```python
from build123d import *

# Parameters (mm, degrees)
SKETCH1_W           = 100
SKETCH1_H           = 20
BOSS_EXTRUDE1_DEPTH = 7
SKETCH2_W           = 16
SKETCH2_H           = 8.428142516
CUT_EXTRUDE1_DEPTH  = 101
SKETCH3_W           = 100
SKETCH3_H           = 62
BOSS_EXTRUDE2_DEPTH = 30
SKETCH4_W           = 88
SKETCH4_H           = 56.5
CUT_EXTRUDE2_DEPTH  = 27.5
SKETCH5_W           = 7.686328358
SKETCH5_H           = 52.5
CUT_EXTRUDE3_DEPTH  = 7
SKETCH6_W           = 27.5
SKETCH6_H           = 13
CUT_EXTRUDE4_DEPTH  = 3
SKETCH7_W           = 58
SKETCH7_H           = 2.3
CUT_EXTRUDE5_DEPTH  = 23
CUT_EXTRUDE6_DEPTH  = 23
SKETCH10_W          = 78.288889142
SKETCH10_H          = 1.311621563
CUT_EXTRUDE7_DEPTH  = 2
FILLET2_R           = 5


with BuildPart() as part:
    # Sketch1 → Boss-Extrude1 (new body)
    with BuildSketch(Plane(origin=(0, 0, 0), x_dir=(1, 0, 0), z_dir=(0, 1, 0))):
        with Locations((-50, 10)):
            Rectangle(SKETCH1_W, SKETCH1_H)
    extrude(amount=BOSS_EXTRUDE1_DEPTH)

    # Sketch2 → Cut-Extrude1 (cut, through all)
    with BuildSketch(Plane.ZY.offset(100)):
        with Locations((-10, 0)):
            Rectangle(SKETCH2_W, SKETCH2_H)
    extrude(amount=-CUT_EXTRUDE1_DEPTH, mode=Mode.SUBTRACT)

    # Sketch3 → Boss-Extrude2 (add)
    with BuildSketch(Plane(origin=(0, 0, -20), x_dir=(-1, 0, 0), z_dir=(0, 0, -1))):
        with Locations((50, -24)):
            Rectangle(SKETCH3_W, SKETCH3_H)
    extrude(amount=BOSS_EXTRUDE2_DEPTH)

    # Sketch4 → Cut-Extrude2 (cut)
    with BuildSketch(Plane(origin=(0, 0, -50), x_dir=(-1, 0, 0), z_dir=(0, 0, -1))):
        with Locations((50, -24)):
            Rectangle(SKETCH4_W, SKETCH4_H)
    extrude(amount=-CUT_EXTRUDE2_DEPTH, mode=Mode.SUBTRACT)

    # Sketch5 → Cut-Extrude3 (cut, through all)
    with BuildSketch(Plane(origin=(-94, 0, 0), x_dir=(0, 0, -1), z_dir=(1, 0, 0))):
        with Locations((35.043164179, -24)):
            Rectangle(SKETCH5_W, SKETCH5_H)
    extrude(amount=-CUT_EXTRUDE3_DEPTH, mode=Mode.SUBTRACT)

    # Sketch6 → Cut-Extrude4 (cut)
    with BuildSketch(Plane.ZY.offset(6)):
        with Locations((-36.25, -24)):
            Rectangle(SKETCH6_W, SKETCH6_H)
    extrude(amount=-CUT_EXTRUDE4_DEPTH, mode=Mode.SUBTRACT)

    # Sketch7 → Cut-Extrude5 (cut)
    with BuildSketch(Plane(origin=(0, 0, -50), x_dir=(-1, 0, 0), z_dir=(0, 0, -1))):
        with Locations((35, -53.4)):
            Rectangle(SKETCH7_W, SKETCH7_H)
    extrude(amount=-CUT_EXTRUDE5_DEPTH, mode=Mode.SUBTRACT)

    # Sketch9 → Cut-Extrude6 (cut)
    with BuildSketch(Plane(origin=(0, -52.25, 0), x_dir=(1, 0, 0), z_dir=(0, 1, 0))):
        Polygon((-37.960647242, 38.5), (-64, 38.5), (-64, 33.5), (-37.960647242, 33.5), (-6.413001969, 33.5), (-6.413001969, 38.5), align=None)
    extrude(amount=-CUT_EXTRUDE6_DEPTH, mode=Mode.SUBTRACT)

    # Sketch10 → Cut-Extrude7 (cut)
    with BuildSketch(Plane(origin=(0, 7, 0), x_dir=(1, 0, 0), z_dir=(0, 1, 0))):
        with Locations((-50, 46.502804438)):
            Rectangle(SKETCH10_W, SKETCH10_H)
    cut_extrude7 = extrude(amount=-CUT_EXTRUDE7_DEPTH, mode=Mode.SUBTRACT)

    # Mirror1: Cut-Extrude7 across plane
    add(cut_extrude7.mirror(Plane.ZX.offset(-24)), mode=Mode.SUBTRACT)

    # Fillet2
    fillet2_edges = [part.edges().sort_by_distance(p)[0] for p in [
        (-50, 7, 0),
    ]]
    fillet(fillet2_edges, radius=FILLET2_R)


solid = part.part
```
Part model, mm, in its own coordinate system. A direction names the side the tool comes from. Round coordinates to 2 decimals unless told otherwise and drop trailing zeros. Order: outer loops, then holes, each group sorted by start corner. A loop starts at its lowest first (then second) coordinate and runs counter-clockwise, first axis right, second up. Notation, with made-up numbers: M -14,-26 L 30,-26 A9 cw 30,-11 Z; hole C -12,-20 d3. An arc over 180 degrees is marked long. Put each result on its own line as item: value. Start each with the question number.
1. Slice it at C-C on z = -44.5. List the corners of the cut face in (x, y), then the cut area to 3 significant figures.
2. Slice it at D-D on x = -78. List the corners of the cut face in (y, z).
3. Slice it at B-B on y = -20. List the corners of the cut face in (x, z).
4. Drop flat-ended pins along their axis: pin 1 (1.3 mm diameter, centred on x = -52.5, y = 1, fed in from -Z); pin 2 (2 mm diameter, centred on x = -87.5, z = -12, fed in from -Y); pin 3 (6 mm diameter, centred on x = -83, y = -13, fed in from +Z). Give the stop position or say it passes through.
5. Two-plate mould, pull along Z, no slides. Class faces 5 (the face through (-53, 6, -50)), 6 (the face through (-51, 0, -1)), 7 (the face through (-97, -24, -38.886)), 8 (the face through (-51, 2, -2)): +Z half, -Z half, draft (parallel to the pull), parting line (faces both ways), or undercut.
6. Tool access for faces 1 (the face through (-51, 4.214, -10)), 2 (the face through (-68, -54, -47.159)), 3 (the face through (-49, 4.25, -36)), 4 (the face through (-49, -27, -20)): list every direction of +Z, -Z, +X, -X, +Y, -Y with a clear straight run to the whole face (end or side of a thin tool).
7. Slice it at A-A on x = -28. State how many separate pieces and enclosed holes the cut face has, then the cut area to 3 significant figures.
8. Drill centre lines: probe 1 along Y at (x, z) = (-88.5, -36); probe 2 along Y at (x, z) = (-25, -39.5); probe 3 along X at (y, z) = (3, -39). Where is each one in solid material? Low to high. Write a range as [from, to].
Findings:
1. outline: M -100,-55 L 0,-55 L 0,7 L -100,7 Z; hole M -94,-52.25 L -64,-52.25 L -64,-54.55 L -6,-54.55 L -6,-30.5 L -3,-30.5 L -3,-17.5 L -6,-17.5 L -6,4.25 L -94,4.25 Z
1. area: 1,060 mm2
2. outline: M -55,-50 L -52.25,-50 L -52.25,-22.5 L 4.25,-22.5 L 4.25,-50 L 7,-50 L 7,-47.16 L 5,-47.16 L 5,-45.85 L 7,-45.85 L 7,-5 A5 ccw 2,0 L 0,0 L 0,-2 L 4.21,-2 L 4.21,-18 L 0,-18 L 0,-20 L -55,-20 L -55,-45.85 L -53,-45.85 L -53,-47.16 L -55,-47.16 Z
3. outline: M -100,-50 L -94,-50 L -94,-38.89 L -100,-38.89 Z; M -100,-31.2 L -94,-31.2 L -94,-22.5 L -3,-22.5 L -3,-50 L 0,-50 L 0,-20 L -100,-20 Z
4. pin 1: z = -22.5
4. pin 2: y = 4.21
4. pin 3: z = -20
5. face 5: -Z half
5. face 6: draft
5. face 7: undercut
5. face 8: undercut
6. face 1: +X, -X, -Y
6. face 2: -Y
6. face 3: -Z
6. face 4: +Z, +X, -X, -Y
7. separate pieces: 3
7. enclosed holes: 0
7. area: 315 mm2
8. probe 1: [-55, -52.25], [4.25, 7]
8. probe 2: [-55, -54.55], [4.25, 7]
8. probe 3: [-100, -94], [-6, 0]
